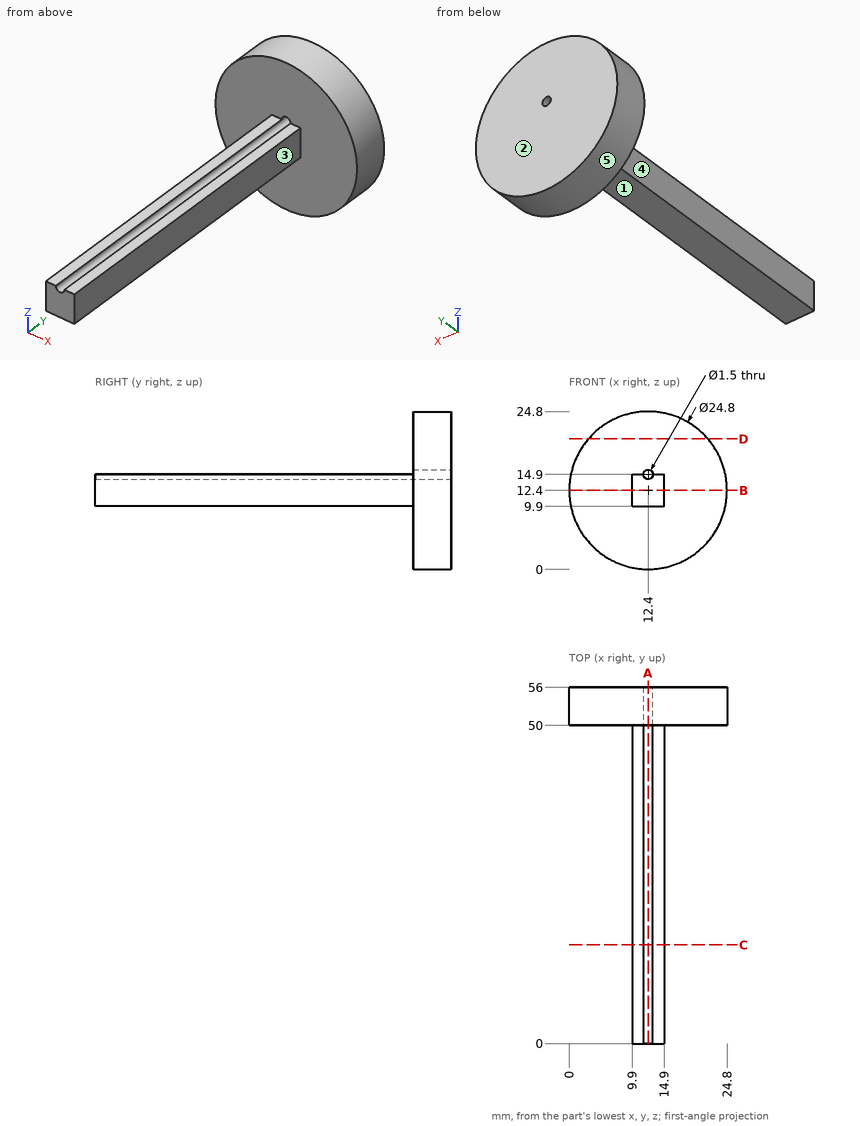
Design review of the part shown in the three views and the two pictorial views. Dimensions are in mm from the part's minimum x, y and z. A direction names the side the tool comes from. Round coordinates to 2 decimals unless told otherwise and drop trailing zeros. Write each loop counter-clockwise with the first axis right and the second up, starting at its lowest first coordinate (ties: lowest second). Pieces come first, ordered by that corner, then holes.
Item 1: For pin 1 Ø1.9 at (x, y) = (11, 25) entering from +Z; pin 2 Ø1 at (x, z) = (15, 16.5) entering from -Y; pin 3 Ø4 at (y, z) = (34, 11.5) entering from +X, all flat-tipped, find the tip position at first contact; note any pin that passes through.
Item 2: Wall thickness on L1, parallel to Z at x = 10.25, y = 12; L2, parallel to Y at x = 22, z = 13.75; L3, parallel to Z at x = 12.4, y = 13: over which ranges is each line inside the solid? List them lowest first.
Item 3: Consider section B-B on z = 12.4. Give the boundary of the cut face in (x, y), and give its area (3 significant figures).
Item 4: For the marked faces 1, 2, 3, 4 and 5, list the 3-axis set-ups (+Z, -Z, +X, -X, +Y, -Y) from which the entire face can be reached by the end or side of a thin tool; tool diameter is ignored.
Item 5: Consider section D-D on z = 20.5. Give the boundary of the cut face in (x, y), and give its area (3 significant figures).
Item 6: Consider section C-C on y = 15.5. Give the boundary of the cut face in (x, z).
Item 7: Consider section A-A on x = 12.4. Give the boundary of the cut face in (y, z).
Check values:
1. pin 1: stops at z = 14.9
1. pin 2: stops at y = 50
1. pin 3: stops at x = 14.9
2. L1: z = 9.9 to 14.9
2. L2: y = 50 to 56
2. L3: z = 9.9 to 14.15
3. outline: (0, 50) - (9.9, 50) - (9.9, 0) - (14.9, 0) - (14.9, 50) - (24.8, 50) - (24.8, 56) - (0, 56) - close
3. area: 399 mm2
4. face 1: -Z, +X, -X, -Y
4. face 2: +Z, -Z, +X, -X, +Y
4. face 3: +Z, -Z, +X, -Y
4. face 4: +Z, -Z, -X, -Y
4. face 5: +Y, -Y
5. outline: (3.01, 50) - (21.79, 50) - (21.79, 56) - (3.01, 56) - close
5. area: 113 mm2
6. outline: (9.9, 9.9) - (14.9, 9.9) - (14.9, 14.9) - (13.15, 14.9) arc R0.75 cw to (11.65, 14.9) - (9.9, 14.9) - close
7. outline: (0, 9.9) - (50, 9.9) - (50, 0) - (56, 0) - (56, 14.15) - (0, 14.15) - close; (50, 15.65) - (56, 15.65) - (56, 24.8) - (50, 24.8) - close
